```python
from build123d import *

# Parameters (mm, degrees)
BOSS_EXTRU_1_START           = 10
ESQUISSE1_R                  = 7.5
BOSS_EXTRU_1_DEPTH           = 120
BOSS_EXTRU_2_START           = 10
BOSS_EXTRU_2_DEPTH           = 20
R_P_TITION_CIRCULAIRE1_COUNT = 3


with BuildPart() as part:
    # Esquisse1 → Boss.-Extru.1 (new body)
    with BuildSketch(Plane(origin=(0, 0, 0), x_dir=(1, 0, 0), z_dir=(0, 1, 0)).offset(BOSS_EXTRU_1_START)):
        with Locations(Location((0, 0, 0), (0, 0, 90))):
            Circle(ESQUISSE1_R)
    extrude(amount=BOSS_EXTRU_1_DEPTH)

    # Esquisse3 → Boss.-Extru.2 (add)
    with BuildSketch(Plane.XZ.offset(-10).offset(BOSS_EXTRU_2_START)):
        with BuildLine():
            Line((3.621916752, -6.567474327), (-3.621916752, -6.567474327))
            Line((-3.621916752, -6.567474327), (-3.621916752, -11.25))
            ThreePointArc((-3.621916752, -11.25), (0, -12.713519057), (3.621916752, -11.25))
            Line((3.621916752, -11.25), (3.621916752, -6.567474327))
        make_face()
    boss_extru_2 = extrude(amount=-BOSS_EXTRU_2_DEPTH)

    # Répétition circulaire1: Boss.-Extru.2 ×3 about axis
    r_p_tition_circulaire1_axis = Axis((0, 0, 0), (0, 1, 0))
    for i in range(1, R_P_TITION_CIRCULAIRE1_COUNT):
        add(boss_extru_2.rotate(r_p_tition_circulaire1_axis, i * 360 / R_P_TITION_CIRCULAIRE1_COUNT))


solid = part.part
```
The model under review builds one solid part; all positions refer to its coordinate system, in mm. A direction names the side the tool comes from. Coordinates: 2 decimals unless noted, no trailing zeros. Write each loop counter-clockwise with the first axis right and the second up, starting at its lowest first coordinate (ties: lowest second). Pieces come first, ordered by that corner, then holes.
1) We need section A-A on x = 0. State the section outline as (y, z) points, then the cut area to 3 significant figures.
2) We need section B-B on y = 82.5. State the section outline as (x, z) points.
3) The part is to be moulded in two halves that separate along X. For faces 6 (the face through (0, 10, 1)), 7 (the face through (-10.98, 9.86, 6.41)), 8 (the face through (9.498, 9.86, 1.301)), say which applies: pulls with the +X half, pulls with the -X half, needs draft (parallel to the pull), parting line crosses it, or undercut.
4) Machinability: for faces 1 (the face through (3.622, 10, -9)), 2 (the face through (5.66, 4.93, 3.33)), 3 (the face through (-6.324, 69.16, -4.032)), 4 (the face through (-5.876, 9.86, 7.575)), 5 (the face through (0, 5, -6.567)), which of the approach directions +Z, -Z, +X, -X, +Y, -Y give a long, thin tool a straight path to every point of the face, cutting with its end or side? Answer none if there is none.
5) To check wall thickness, follow probe 1 along Y at (x, z) = (-3.25, -11); probe 2 along X at (y, z) = (24, 0.25); probe 3 along Y at (x, z) = (-0.25, 2.25). State the ranges of each line that lie inside material, in increasing order.
6) Clearance check with flat-ended pins moving along their axes: pin 1 Ø4 at (x, z) = (0, 2) entering from -Y; pin 2 Ø6 at (x, y) = (1.5, 13) entering from +Z; pin 3 Ø5 at (x, y) = (6.5, 59.5) entering from -Z; pin 4 Ø5 at (x, z) = (0, -8.5) entering from +Y. State where each tip first meets the part, or that it passes through.
Answer list:
1. outline: (0, -12.71) - (20, -12.71) - (20, -7.5) - (130, -7.5) - (130, 7.5) - (10, 7.5) - (10, -6.57) - (0, -6.57) - close
1. area: 1,910 mm2
2. outline: circle Ø15 at (0, 0)
3. face 6: undercut
3. face 7: pulls with the -X half
3. face 8: pulls with the +X half
4. face 1: -Z, +X, +Y, -Y
4. face 2: -Z, -Y
4. face 3: +Y
4. face 4: +Z, +Y, -Y
4. face 5: +Z, +X, -X, -Y
5. probe 1: y = 0 to 20
5. probe 2: x = -7.5 to 7.5
5. probe 3: y = 10 to 130
6. pin 1: stops at y = 10
6. pin 2: stops at z = 7.5
6. pin 3: stops at z = -6.34
6. pin 4: stops at y = 130
